from build123d import *

# Parameters (mm, degrees)
SKETCH1_R           = 12.5
SKETCH1_R_2         = 8
BOSS_EXTRUDE1_DEPTH = 2.5
SKETCH3_R           = 20
SKETCH3_R_2         = 8
BOSS_EXTRUDE3_DEPTH = 5
CHAMFER2_SIZE       = 1
SKETCH4_W           = 11
SKETCH4_H           = 7.5
BOSS_EXTRUDE4_DEPTH = 3


with BuildPart() as part:
    # Sketch1 → Boss-Extrude1 (new body)
    with BuildSketch(Plane.XY):
        Circle(SKETCH1_R)
        Circle(SKETCH1_R_2, mode=Mode.SUBTRACT)
    extrude(amount=BOSS_EXTRUDE1_DEPTH)

    # Sketch3 → Boss-Extrude3 (add)
    with BuildSketch(Plane(origin=(0, 0, 0), x_dir=(-1, 0, 0), z_dir=(0, 0, -1))):
        Circle(SKETCH3_R)
        Circle(SKETCH3_R_2, mode=Mode.SUBTRACT)
    extrude(amount=BOSS_EXTRUDE3_DEPTH)

    # Chamfer2
    chamfer2_edges = [part.edges().sort_by_distance(p)[0] for p in [
        (20, 0, 0),
        (20, 0, -5),
    ]]
    chamfer(chamfer2_edges, length=CHAMFER2_SIZE)

    # Sketch4 → Boss-Extrude4 (add)
    with BuildSketch(Plane(origin=(0, -6, 0), x_dir=(-1, 0, 0), z_dir=(0, 1, 0))):
        with Locations((0, -1.25)):
            Rectangle(SKETCH4_W, SKETCH4_H)
    extrude(amount=-BOSS_EXTRUDE4_DEPTH)


solid = part.part
Work out the finished part from the listing and answer in its coordinate system (mm). A direction names the side the tool comes from. Coordinates: 2 decimals unless noted, no trailing zeros. Write each loop counter-clockwise with the first axis right and the second up, starting at its lowest first coordinate (ties: lowest second). Pieces come first, ordered by that corner, then holes. Notation, with made-up numbers: M -30.5,34 L 19.5,34 A28 ccw 19.5,61 Z; hole C 20.5,78 d9. An arc over 180 degrees is marked long. Write item = value, one per line.
1. The part is cut by section B-B (x = 0). Determine the outline of the cut face in (y, z).
Solution:
outline = M -20,-4 L -19,-5 L -6,-5 L -6,2.5 L -12.5,2.5 L -12.5,0 L -19,0 L -20,-1 Z; M 8,-5 L 19,-5 L 20,-4 L 20,-1 L 19,0 L 12.5,0 L 12.5,2.5 L 8,2.5 Z
2. For faces 1 (the face through (4.336, -19.524, -2.479)), 2 (the face through (-12.4, -4, 0)), determine the directions among +Z, -Z, +X, -X, +Y, -Y from which every point of the face is accessible in a straight line to the end or side of a thin tool.
Solution:
face_1 = +Z, -Z
face_2 = +Z
3. Straight lines are drawn through the part: line 1 (Y direction, x = 0, z = 1); line 2 (Z direction, x = 12.5, y = -5.5); line 3 (Y direction, x = -6, z = -3.75). For each, find the intervals that lie inside material, in ascending order. Write a range as from..to.
Solution:
line_1 = -12.5..-6, 8..12.5
line_2 = -5..0
line_3 = -19.08..-5.29, 5.29..19.08
4. Determine the mould class of faces 3 (the face through (11.923, 3.755, 1.232)), 4 (the face through (-8.2, 0.3, -5)), 5 (the face through (0, -6, -1)) for opening direction X: released by +X, released by -X, zero draft, split by the parting line, or undercut.
Solution:
face_3 = split by the parting line
face_4 = zero draft
face_5 = undercut
5. The part is cut by section A-A (y = 0). Determine the outline of the cut face in (x, z), then the cut area to 4 significant figures.
Solution:
outline = M -20,-4 L -19,-5 L -8,-5 L -8,2.5 L -12.5,2.5 L -12.5,0 L -19,0 L -20,-1 Z; M 8,-5 L 19,-5 L 20,-4 L 20,-1 L 19,0 L 12.5,0 L 12.5,2.5 L 8,2.5 Z
area = 140.5 mm2
6. The part is cut by section C-C (z = -3.25). Determine the outline of the cut face in (x, y), then the cut area to 3 significant figures.
Solution:
outline = C 0,0 d40; hole M -5.29,-6 L 5.29,-6 A8 ccw long Z
area = 1,070 mm2
7. Flat-ended cylindrical pins translate along their axes: pin 1 (1 mm diameter, centred on y = 9, z = -2, fed in from -X); pin 2 (6 mm diameter, centred on x = -9.5, y = -15, fed in from +Z); pin 3 (4 mm diameter, centred on x = 2, z = -2.5, fed in from +Y). Find the tip coordinate at first contact, or state that the pin passes through.
Solution:
pin_1 = -18.1
pin_2 = 0
pin_3 = 20
